Source: three-view drawing plus pictorial views. Frame: mm from the lowest corner of the part. A direction names the side the tool comes from. Give positions to 0.01 mm unless a question says otherwise; leave off trailing zeros. Order: outer loops, then holes, each group sorted by start corner. A loop starts at its lowest first (then second) coordinate and runs counter-clockwise, first axis right, second up. Notation, with made-up numbers: M -27.75,89.25 L -13.75,89.25 A27 cw -13.75,109.25 Z; hole C 43.25,32.5 d3. An arc over 180 degrees is marked long. One line per question, with ' | ' between items. Start each with the question number.
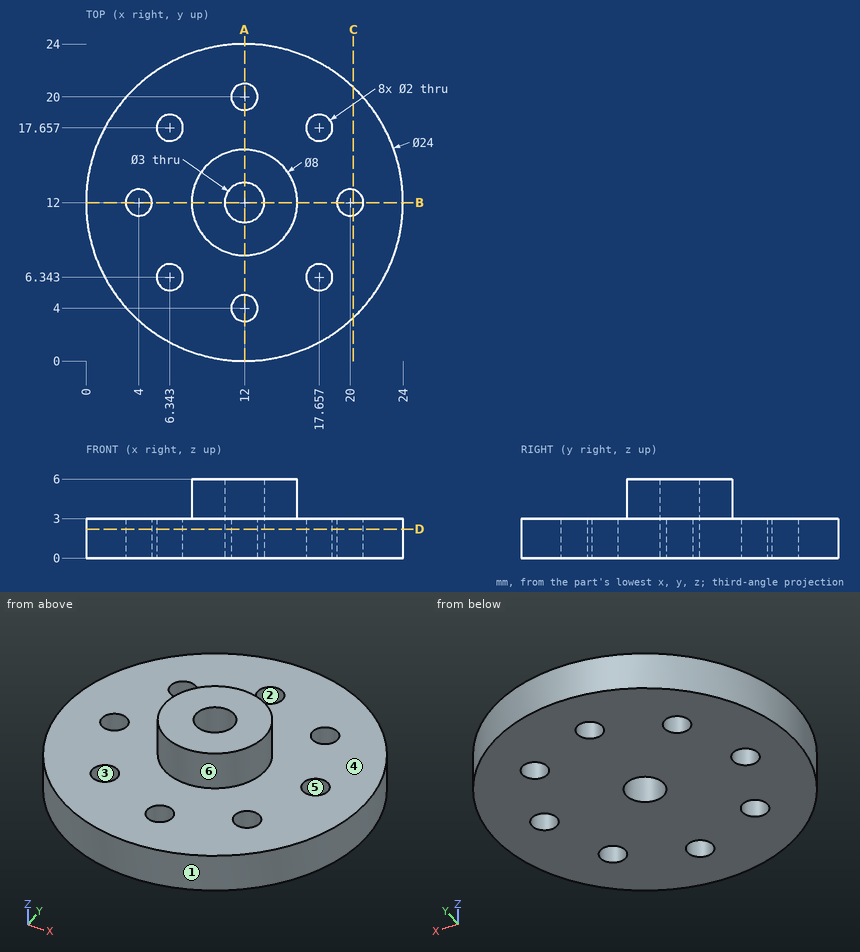
Item 1: Cut plane A-A on x = 12. Return the cut outline in (y, z).
Item 2: Cut plane C-C on x = 20.25. Return the cut outline in (y, z), and give its area (3 significant figures).
Item 3: Pin query (flat end, axial travel): pin 1 Ø1.2 at (x, y) = (6.34, 6.34) entering from +Z; pin 2 Ø1.5 at (x, y) = (15, 8) entering from -Z; pin 3 Ø3 at (x, y) = (17.66, 6.34) entering from +Z; pin 4 Ø3 at (x, z) = (18.5, 3) entering from -Y. Return the tip coordinate at first contact, or that it passes through.
Item 4: Cut plane D-D on z = 2.2. Count the separate pieces of the cut face and the enclosed holes in it, and give its area (3 significant figures).
Item 5: Mould query, pull axis Y, two halves, no side actions, for the marked faces 1, 2, 3 and 4. Classes: pulls with the +Y half, pulls with the -Y half, needs draft (parallel to the pull), parting line crosses it, or undercut.
Item 6: Reachability of the marked faces 5 and 6 from +Z, -Z, +X, -X, +Y, -Y: full face, straight path, thin tool, end or side. Return the list, or none.
Item 7: Line query: line 1 (Y direction, x = 17.25, z = 2.8); line 2 (Z direction, x = 3.75, y = 6.25); line 3 (Y direction, x = 21.75, z = 1.1) (1 decimal). Output: solid intervals per line, ascending.
Results are:
1) outline: M 0,0 L 3,0 L 3,3 L 0,3 Z; M 5,0 L 10.5,0 L 10.5,6 L 8,6 L 8,3 L 5,3 Z; M 13.5,0 L 19,0 L 19,3 L 16,3 L 16,6 L 13.5,6 Z; M 21,0 L 24,0 L 24,3 L 21,3 Z
2) outline: M 3.29,0 L 11.03,0 L 11.03,3 L 3.29,3 Z; M 12.97,0 L 20.71,0 L 20.71,3 L 12.97,3 Z | area: 46.5 mm2
3) pin 1: passes through | pin 2: stops at z = 0 | pin 3: stops at z = 3 | pin 4: stops at y = 1.09
4) separate pieces: 1 | enclosed holes: 9 | area: 420 mm2
5) face 1: parting line crosses it | face 2: undercut | face 3: undercut | face 4: needs draft
6) face 5: +Z, -Z | face 6: +Z
7) line 1: y = 1.21 to 5.43, 7.26 to 16.74, 18.57 to 22.79 | line 2: z = 0 to 3 | line 3: y = 5 to 19
